Check sheet for the modelled part. Datum: model origin and axes. Units: mm. Face numbers are marked on the shaded views. A direction names the side the tool comes from. Round coordinates to 2 decimals unless told otherwise and drop trailing zeros. Order: outer loops, then holes, each group sorted by start corner. A loop starts at its lowest first (then second) coordinate and runs counter-clockwise, first axis right, second up. Notation, with made-up numbers: M -25.5,42 L 30.5,42 A29 ccw 30.5,74 Z; hole C 85,52.5 d6. An arc over 180 degrees is marked long. One line per item, written item: value. Start each with the question number.
(1) Cross-section at A-A, the plane z = 19. Enter the section's corners in (x, y), and give its area (3 significant figures).
(2) Cross-section at B-B, the plane x = 5. Enter the section's corners in (y, z).
(3) Access from +Z, -Z, +X, -X, +Y, -Y to the whole of each face (thin tool, end or side, straight path). Record for the marked faces 1 and 2.
(4) Release check for a two-part mould opening along Y. For the marked faces 3, 4, 5 and 6 record: released by +Y, released by -Y, zero draft, split by the parting line, or undercut.
(5) Cross-section at C-C, the plane y = 0. Enter the section's corners in (x, z).
(6) Thickness scan on L1, parallel to X at y = 12.5, z = 62; L2, parallel to Z at x = -15.1, y = 0. Record the ranges inside material, lowest first.
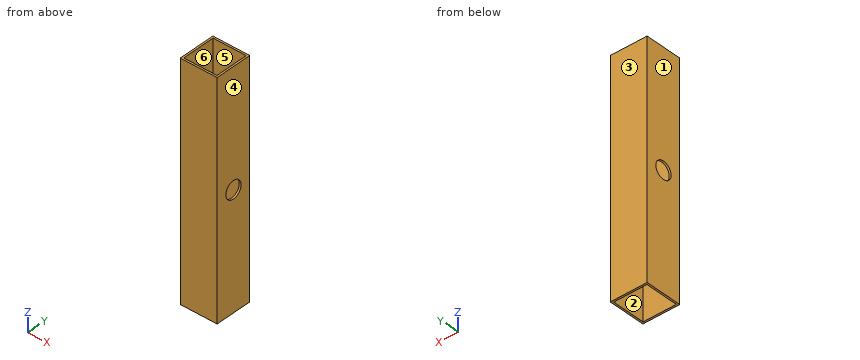
Autodesk Inventor part; units mm, degrees
ref_plane "作業平面1" through (16, -16, 100) normal (1, 0, 0) x (0, 0, -1)
ref_plane "YZ Plane" through (0, 0, 0) normal (1, 0, 0) x (0, 1, 0)
ref_plane "XZ Plane" through (0, 0, 0) normal (0, 1, 0) x (-1, 0, 0)
sketch "スケッチ1" plane through (0, 0, 0) normal (0, 0, 1) x (1, 0, 0)
  line L0 (-16, -16) -> (16, -16)
  line L1 (16, -16) -> (16, 16)
  line L2 (16, 16) -> (-16, 16)
  line L3 (-16, 16) -> (-16, -16)
  line L4 (-16, -16) -> (16, 16) construction
  line L5 (16, -16) -> (-16, 16) construction
  line L6 (-14.4, 14.4) -> (14.4, 14.4)
  line L7 (14.4, 14.4) -> (14.4, -14.4)
  line L8 (14.4, -14.4) -> (-14.4, -14.4)
  line L9 (-14.4, -14.4) -> (-14.4, 14.4)
  point P0 (0, 0)
  dimension "d0" = 32
  dimension "d1" = 32
  dimension "d2" = 1.6
extrude "押し出し1" add sketch "スケッチ1" along normal mid plane 200
ref_plane "作業平面1" through (16, -16, 100) normal (1, 0, 0) x (0, 0, -1)
sketch "スケッチ2" plane through (16, -16, 100) normal (1, 0, 0) x (0, 0, -1)
  point P0 (100, 16)
  point P1 (100, 16)
hole "穴1" at (16, 0, 0) direction (-1, 0, 0) diameter 15 end through all
properties part number "Pipe横"
Values found:
1. outline: M -16,-16 L 16,-16 L 16,16 L -16,16 Z; hole M -14.4,-14.4 L 14.4,-14.4 L 14.4,14.4 L -14.4,14.4 Z
1. area: 195 mm^2
2. outline: M -16,-100 L -14.4,-100 L -14.4,100 L -16,100 Z; M 14.4,-100 L 16,-100 L 16,100 L 14.4,100 Z
3. face 1: +Z, -Z, -X, +Y, -Y
3. face 2: +Z, -Z
4. face 3: released by +Y
4. face 4: zero draft
4. face 5: undercut
4. face 6: undercut
5. outline: M -16,-100 L -14.4,-100 L -14.4,-7.5 L -16,-7.5 Z; M -16,7.5 L -14.4,7.5 L -14.4,100 L -16,100 Z; M 14.4,-100 L 16,-100 L 16,-7.5 L 14.4,-7.5 Z; M 14.4,7.5 L 16,7.5 L 16,100 L 14.4,100 Z
6. L1: -16 to -14.4, 14.4 to 16
6. L2: -100 to -7.5, 7.5 to 100
